```python
from build123d import *

# Parameters (mm, degrees)
SKETCH_1_W          = 86
SKETCH_1_H          = 174
SKETCH_1_W_2        = 50
SKETCH_1_H_2        = 25
SKETCH_1_H_3        = 55
SKETCH_1_W_3        = 76
SKETCH_1_H_4        = 43
EXTRUDE_1_DEPTH     = 5
SKETCH_4_W          = 68.7
SKETCH_4_H          = 115
SKETCH_4_W_2        = 64.7
SKETCH_4_H_2        = 37
SKETCH_4_H_3        = 70
EXTRUDE_2_DEPTH     = 10
SKETCH_5_R          = 0.75
CUT_EXTRUDE_1_DEPTH = 122.783619588
SKETCH_7_W          = 15
SKETCH_7_H          = 8
SKETCH_7_W_2        = 26
SKETCH_7_W_3        = 5
SKETCH_7_H_2        = 10
SKETCH_7_H_3        = 12.119700025
SKETCH_7_W_4        = 6
SKETCH_7_H_4        = 5
SKETCH_7_W_5        = 7
SKETCH_7_H_5        = 21
CUT_EXTRUDE_2_DEPTH = 2
SKETCH_8_R          = 0.75
CUT_EXTRUDE_3_DEPTH = 2
CUT_EXTRUDE_START   = -84
SKETCH_8_3_R        = 0.75
CUT_EXTRUDE_4_DEPTH = 2
SKETCH_9_R          = 0.75
SKETCH_9_W          = 50
SKETCH_9_H          = 25
SKETCH_9_W_2        = 76
SKETCH_9_H_2        = 43
CUT_EXTRUDE_5_DEPTH = 123.295748086


with BuildPart() as part:
    # 草图1 → 凸台-拉伸1 (new body)
    with BuildSketch(Plane(origin=(0, 0, 0), x_dir=(1, 0, 0), z_dir=(0, 1, 0))):
        with Locations((0, -26.5)):
            Rectangle(SKETCH_1_W, SKETCH_1_H)
        with Locations((0, -38)):
            Rectangle(SKETCH_1_W_2, SKETCH_1_H_2, mode=Mode.SUBTRACT)
        with Locations((0, 23)):
            Rectangle(SKETCH_1_W_2, SKETCH_1_H_3, mode=Mode.SUBTRACT)
        with Locations((0, -87)):
            Rectangle(SKETCH_1_W_3, SKETCH_1_H_4, mode=Mode.SUBTRACT)
    extrude(amount=EXTRUDE_1_DEPTH)

    # 草图4 → 凸台-拉伸2 (add)
    with BuildSketch(Plane(origin=(0, 5, 0), x_dir=(1, 0, 0), z_dir=(0, 1, 0))):
        Rectangle(SKETCH_4_W, SKETCH_4_H)
        with Locations((0, -37)):
            Rectangle(SKETCH_4_W_2, SKETCH_4_H_2, mode=Mode.SUBTRACT)
        with Locations((0, 20.5)):
            Rectangle(SKETCH_4_W_2, SKETCH_4_H_3, mode=Mode.SUBTRACT)
    extrude(amount=EXTRUDE_2_DEPTH)

    # 草图5 → 切除-拉伸1 (cut, through all)
    with BuildSketch(Plane(origin=(0, 5, 0), x_dir=(1, 0, 0), z_dir=(0, 1, 0))):
        with Locations(Location((-39, 20.5, 0), (0, 0, 270))):
            Circle(SKETCH_5_R)
        with Locations(Location((39, 20.5, 0), (0, 0, 270))):
            Circle(SKETCH_5_R)
        with Locations(Location((-39, -32.5, 0), (0, 0, 270))):
            Circle(SKETCH_5_R)
        with Locations(Location((39, -32.5, 0), (0, 0, 270))):
            Circle(SKETCH_5_R)
        with Locations(Location((-40.1427775, -60.35, 0), (0, 0, 270))):
            Circle(SKETCH_5_R)
        with Locations(Location((40.1427775, -60.35, 0), (0, 0, 270))):
            Circle(SKETCH_5_R)
        with Locations(Location((-40.1427775, -110.530299975, 0), (0, 0, 270))):
            Circle(SKETCH_5_R)
        with Locations(Location((40.1427775, -110.530299975, 0), (0, 0, 270))):
            Circle(SKETCH_5_R)
        with Locations(Location((-40.5, 57.5, 0), (0, 0, 270))):
            Circle(SKETCH_5_R)
        with Locations(Location((-40.5, -38, 0), (0, 0, 270))):
            Circle(SKETCH_5_R)
        with Locations(Location((-40.5, -85.5, 0), (0, 0, 270))):
            Circle(SKETCH_5_R)
        with Locations(Location((40.5, 57.5, 0), (0, 0, 270))):
            Circle(SKETCH_5_R)
        with Locations(Location((40.5, -38, 0), (0, 0, 270))):
            Circle(SKETCH_5_R)
        with Locations(Location((40.5, -85.5, 0), (0, 0, 270))):
            Circle(SKETCH_5_R)
        with Locations(Location((-40.5, -4.5, 0), (0, 0, 270))):
            Circle(SKETCH_5_R)
        with Locations(Location((40.5, -4.5, 0), (0, 0, 270))):
            Circle(SKETCH_5_R)
    extrude(amount=-CUT_EXTRUDE_1_DEPTH, mode=Mode.SUBTRACT)

    # 草图7 → 切除-拉伸2 (cut)
    with BuildSketch(Plane(origin=(0, 5, 0), x_dir=(1, 0, 0), z_dir=(0, 1, 0))):
        with Locations((-24.5, -61.5)):
            Rectangle(SKETCH_7_W, SKETCH_7_H)
        with Locations((0, -61.5)):
            Rectangle(SKETCH_7_W_2, SKETCH_7_H)
        with Locations((-40.5, -78.5)):
            Rectangle(SKETCH_7_W_3, SKETCH_7_H_2)
        with Locations((-40.5, -101.440149988)):
            Rectangle(SKETCH_7_W_3, SKETCH_7_H_3)
        with Locations((-32, -111)):
            Rectangle(SKETCH_7_W_4, SKETCH_7_H_4)
        with Locations((-3, -111)):
            Rectangle(SKETCH_7_W_4, SKETCH_7_H_4)
        with Locations((17.5, -111)):
            Rectangle(SKETCH_7_W_5, SKETCH_7_H_4)
        with Locations((30.5, -111)):
            Rectangle(SKETCH_7_W_5, SKETCH_7_H_4)
        with Locations((40.5, -92)):
            Rectangle(SKETCH_7_W_3, SKETCH_7_H_5)
    extrude(amount=-CUT_EXTRUDE_2_DEPTH, mode=Mode.SUBTRACT)

    # 草图8 → 切除-拉伸3 (cut)
    with BuildSketch(Plane.ZY.offset(43)):
        with Locations((8, 2.5)):
            Circle(SKETCH_8_R)
        with Locations((23, 2.5)):
            Circle(SKETCH_8_R)
        with Locations((52, 2.5)):
            Circle(SKETCH_8_R)
        with Locations((63, 2.5)):
            Circle(SKETCH_8_R)
    extrude(amount=-CUT_EXTRUDE_3_DEPTH, mode=Mode.SUBTRACT)

    # 草图8<3> → 切除-拉伸4 (cut)
    with BuildSketch(Plane.ZY.offset(43).offset(CUT_EXTRUDE_START)):
        with Locations((8, 2.5)):
            Circle(SKETCH_8_3_R)
        with Locations((23, 2.5)):
            Circle(SKETCH_8_3_R)
        with Locations((52, 2.5)):
            Circle(SKETCH_8_3_R)
        with Locations((63, 2.5)):
            Circle(SKETCH_8_3_R)
    extrude(amount=-CUT_EXTRUDE_4_DEPTH, mode=Mode.SUBTRACT)

    # 草图9 → 切除-拉伸5 (cut, through all)
    with BuildSketch(Plane(origin=(0, 0, 0), x_dir=(1, 0, 0), z_dir=(0, 1, 0))):
        Polygon((0, -16.5), (-43, -16.5), (-43, -113.5), (43, -113.5), (43, -16.5), align=None)
        with Locations((-40.5, -38)):
            Circle(SKETCH_9_R, mode=Mode.SUBTRACT)
        with Locations((-39, -32.5)):
            Circle(SKETCH_9_R, mode=Mode.SUBTRACT)
        with Locations((0, -38)):
            Rectangle(SKETCH_9_W, SKETCH_9_H, mode=Mode.SUBTRACT)
        with Locations((40.5, -38)):
            Circle(SKETCH_9_R, mode=Mode.SUBTRACT)
        with Locations((39, -32.5)):
            Circle(SKETCH_9_R, mode=Mode.SUBTRACT)
        with Locations((40.1427775, -60.35)):
            Circle(SKETCH_9_R, mode=Mode.SUBTRACT)
        with Locations((-40.1427775, -110.530299975)):
            Circle(SKETCH_9_R, mode=Mode.SUBTRACT)
        with Locations((-40.5, -85.5)):
            Circle(SKETCH_9_R, mode=Mode.SUBTRACT)
        with Locations((0, -87)):
            Rectangle(SKETCH_9_W_2, SKETCH_9_H_2, mode=Mode.SUBTRACT)
        with Locations((-40.1427775, -60.35)):
            Circle(SKETCH_9_R, mode=Mode.SUBTRACT)
        with Locations((40.1427775, -110.530299975)):
            Circle(SKETCH_9_R, mode=Mode.SUBTRACT)
        with Locations((40.5, -85.5)):
            Circle(SKETCH_9_R, mode=Mode.SUBTRACT)
    extrude(amount=CUT_EXTRUDE_5_DEPTH, mode=Mode.SUBTRACT)


solid = part.part
```
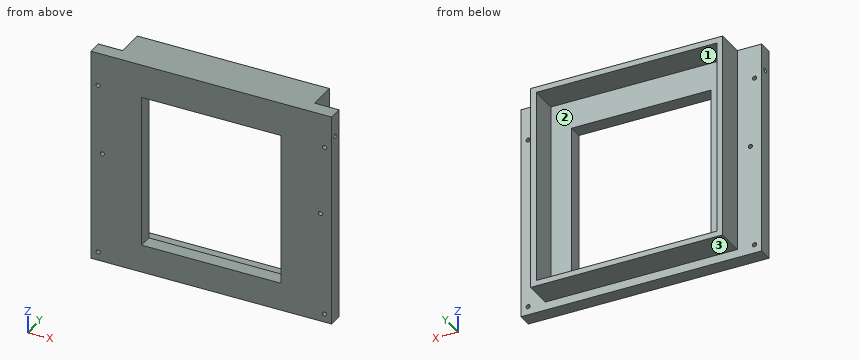
Part model, mm, in its own coordinate system. Face numbers are marked on the shaded views. Round coordinates to 2 decimals unless told otherwise and drop trailing zeros. Order: outer loops, then holes, each group sorted by start corner. A loop starts at its lowest first (then second) coordinate and runs counter-clockwise, first axis right, second up. Notation, with made-up numbers: M 47.5,37 L 70.5,37 A13 ccw 70.5,47 Z; hole C 72.5,-28 d2. An arc over 180 degrees is marked long. Put each result on its own line as item: value. Start each with the question number.
1. Slice it at A-A on z = -32.5. List the corners of the cut face in (x, y), then the cut area to 3 significant figures.
2. Drill centre lines: probe 1 along Z at (x, y) = (40.5, 4.05); probe 2 along X at (y, z) = (3.5, -43.5); probe 3 along X at (y, z) = (7, -26). Where is each one in solid material? Low to high. Write a range as [from, to].
3. Slice it at C-C on y = 9.5. List the corners of the cut face in (x, z), then the cut area to 3 significant figures.
4. Drop flat-ended pins along their axis: pin 1 (2 mm diameter, centred on x = -27.5, y = 12.5, fed in from -Z); pin 2 (8 mm diameter, centred on y = 9.5, z = -18.5, fed in from -X); pin 3 (12 mm diameter, centred on x = 24.5, z = -39.5, fed in from +Y). Give the stop position or say it passes through.
5. Slice it at B-B on x = 31. List the corners of the cut face in (y, z), then the cut area to 3 significant figures.
6. Two-plate mould, pull along X, no slides. Class the marked faces 1, 2 and 3: +X half, -X half, draft (parallel to the pull), parting line (faces both ways), or undercut.
Findings:
1. outline: M -43,0 L -25,0 L -25,5 L -32.35,5 L -32.35,15 L -34.35,15 L -34.35,5 L -43,5 Z; M 25,0 L 43,0 L 43,5 L 34.35,5 L 34.35,15 L 32.35,15 L 32.35,5 L 25,5 Z
1. area: 220 mm2
2. probe 1: [-60.5, -58.25], [-56.75, 3.75], [5.25, 16.5]
2. probe 2: [-43, -25], [25, 43]
2. probe 3: [-34.35, -32.35], [32.35, 34.35]
3. outline: M -34.35,-57.5 L 34.35,-57.5 L 34.35,16.5 L -34.35,16.5 Z; hole M -32.35,-55.5 L 32.35,-55.5 L 32.35,14.5 L -32.35,14.5 Z
3. area: 555 mm2
4. pin 1: z = -57.5
4. pin 2: x = -34.35
4. pin 3: y = 5
5. outline: M 0,-60.5 L 5,-60.5 L 5,-57.5 L 15,-57.5 L 15,-55.5 L 5,-55.5 L 5,14.5 L 15,14.5 L 15,16.5 L 0,16.5 Z
5. area: 425 mm2
6. face 1: undercut
6. face 2: undercut
6. face 3: draft
